from build123d import *

# Parameters (mm, degrees)
F0_R     = 19.05
F1_DEPTH = 50.8
F0_R_2   = 6.857792
F2_DEPTH = 19.05
F3_DEPTH = 19.05
F0_R_3   = 12.7
F4_DEPTH = 38.1


with BuildPart() as f1:
    # F0 (on Top) → F1 (new body)
    with BuildSketch(Plane.XY):
        with BuildLine():
            ThreePointArc((29.102578, -12.692613), (31.081098, -6.482887), (31.75, 0))
            ThreePointArc((31.75, 0), (31.080701, 6.484792), (29.101022, 12.696182))
            ThreePointArc((29.101022, 12.696182), (-0.00495, 31.75), (-29.10498, 12.687106))
            ThreePointArc((-29.10498, 12.687106), (-31.75, -0.005082), (-29.100917, -12.696423))
            ThreePointArc((-29.100917, -12.696423), (0.002078, -31.75), (29.102578, -12.692613))
        make_face()
        Circle(F0_R, mode=Mode.SUBTRACT)
    extrude(amount=F1_DEPTH)

    # F0 (on Top) → F2 (join)
    with BuildSketch(Plane.XY):
        with BuildLine():
            ThreePointArc((-29.100917, -12.696423), (-31.75, -0.005082), (-29.10498, 12.687106))
            Line((-29.10498, 12.687106), (-58.254777, 12.687106))
            Line((-58.254777, 12.687106), (-59.399047, 12.687106))
            ThreePointArc((-59.399047, 12.687106), (-71.52619, -0.135445), (-59.128318, -12.696423))
            Line((-59.128318, -12.696423), (-58.525507, -12.696423))
            Line((-58.525507, -12.696423), (-29.100917, -12.696423))
        make_face()
        with Locations((-58.826912, 0)):
            Circle(F0_R_2, mode=Mode.SUBTRACT)
    extrude(amount=F2_DEPTH)

    # F0 (on Top) → F3 (join)
    with BuildSketch(Plane.XY):
        with BuildLine():
            ThreePointArc((29.101022, 12.696182), (31.080701, 6.484792), (31.75, 0))
            ThreePointArc((31.75, 0), (31.081098, -6.482887), (29.102578, -12.692613))
            Line((29.102578, -12.692613), (74.115909, -12.692613))
            Line((74.115909, -12.692613), (74.982091, -12.692613))
            ThreePointArc((74.982091, -12.692613), (87.248854, 0.060869), (74.860406, 12.696182))
            Line((74.860406, 12.696182), (74.237594, 12.696182))
            Line((74.237594, 12.696182), (29.101022, 12.696182))
        make_face()
        with BuildLine():
            ThreePointArc((74.548989, 6.858), (81.407, -0.000503), (74.547984, -6.858))
            Line((74.547984, -6.858), (46.607984, -6.853861))
            ThreePointArc((46.607984, -6.853861), (39.512576, -0.106876), (46.394271, 6.857956))
            Line((46.394271, 6.857956), (74.548989, 6.858))
        make_face(mode=Mode.SUBTRACT)
    extrude(amount=F3_DEPTH)

    # F0 (on Top) → F4 (join)
    with BuildSketch(Plane.XY):
        Circle(F0_R)
        Circle(F0_R_3, mode=Mode.SUBTRACT)
    extrude(amount=F4_DEPTH)


solid = f1.part
Read the model definition and answer for the solid it produces. Units are mm, in the model's axes. A direction names the side the tool comes from. Coordinates: 2 decimals unless noted, no trailing zeros. Write each loop counter-clockwise with the first axis right and the second up, starting at its lowest first coordinate (ties: lowest second). Pieces come first, ordered by that corner, then holes. Notation, with made-up numbers: (11.5, 1) -> (29.5, 1) arc R21 ccw to (29.5, 18) -> close; hole circle Ø1 at (23, 8). An arc over 180 degrees is marked (long way). Return JSON: item names as keys, results as strings.
(1) Consider line 1 along Y through (x, z) = (0, 44); line 2 along Y through (x, z) = (47, 18.5); line 3 along Z through (x, y) = (-53, -6.5). Determine where each line is inside the solid, lowest interval first. Write a range as from..to.
Answers below:
{"line 1": "-31.75..-19.05, 19.05..31.75", "line 2": "-12.69..-6.85, 6.86..12.7", "line 3": "0..19.05"}
(2) The part is cut by section B-B on z = 28. Give the vertices of the cut face in (x, y).
Answers below:
{"outline": "(29.1, -12.69) arc R31.75 ccw to (31.75, 0) arc R31.75 ccw to (29.1, 12.7) arc R31.75 ccw (long way) to start; hole circle Ø25.4 at (0, 0)"}
(3) Each of these flat-tipped pins is pushed along its axis until it touches: P1, Ø21, axis at x = -44, z = 10, coming from the -Y side; P2, Ø9.5, axis at x = -37.5, z = 13.5, coming from the +Y side; P3, Ø5, axis at x = -45, y = 0.5, coming from the +Z side; P4, Ø1, axis at x = 9, y = -11.5, coming from the -Z side. Where does it stop, or does it pass through?
Answers below:
{"P1": "y = -12.7", "P2": "y = 12.69", "P3": "z = 19.05", "P4": "z = 0"}
(4) The part is cut by section D-D on y = -10. Give the vertices of the cut face in (x, z), then the cut area to 3 significant figures.
Answers below:
{"outline": "(-66.66, 0) -> (-7.83, 0) -> (-7.83, 38.1) -> (-16.21, 38.1) -> (-16.21, 50.8) -> (-30.13, 50.8) -> (-30.13, 19.05) -> (-66.66, 19.05) -> close; (7.83, 0) -> (82.38, 0) -> (82.38, 19.05) -> (30.13, 19.05) -> (30.13, 50.8) -> (16.21, 50.8) -> (16.21, 38.1) -> (7.83, 38.1) -> close", "area": "3,740 mm^2"}
(5) Which of the six approach directions +Z, -Z, +X, -X, +Y, -Y give full straight-line access (tool end or side, diameter ignored) to faces 4 (the cylindrical face through (39.517, -0.259, 9.392)), 5 (the flat face through (-44, 12.687, 9)), 6 (the flat face through (52, 12.696, 9)), 7 (the cylindrical face through (-15.12, -11.59, 44.36))?
Answers below:
{"face 4": "+Z, -Z", "face 5": "+Z, -Z, -X, +Y", "face 6": "+Z, -Z, +X, +Y", "face 7": "+Z"}
(6) The part is cut by section C-C on z = 12. Give the vertices of the cut face in (x, y).
Answers below:
{"outline": "(-59.4, 12.69) arc R12.7 ccw to (-59.13, -12.7) -> (-29.1, -12.7) arc R31.75 ccw to (29.1, -12.69) -> (74.98, -12.69) arc R12.7 ccw to (74.86, 12.7) -> (29.1, 12.7) arc R31.75 ccw to (-29.1, 12.69) -> close; hole circle Ø13.72 at (-58.83, 0); hole circle Ø25.4 at (0, 0); hole (46.39, 6.86) arc R6.86 ccw (long way) to (46.61, -6.85) -> (74.55, -6.86) arc R6.86 ccw to (74.55, 6.86) -> close"}
(7) For a pull along X with two mould halves and no side action, classify faces 1 (the cylindrical face through (-2.75, -12.4, 18.78)), 2 (the flat face through (-11, -7, 0)), 3 (the cylindrical face through (-71.526, 0.138, 9.392)) as pulls with the +X half, pulls with the -X half, needs draft (parallel to the pull), parting line crosses it, or undercut.
Answers below:
{"face 1": "undercut", "face 2": "needs draft", "face 3": "pulls with the -X half"}
(8) The part is cut by section A-A on x = 0. Give the vertices of the cut face in (y, z).
Answers below:
{"outline": "(-31.75, 0) -> (-12.7, 0) -> (-12.7, 38.1) -> (-19.05, 38.1) -> (-19.05, 50.8) -> (-31.75, 50.8) -> close; (12.7, 0) -> (31.75, 0) -> (31.75, 50.8) -> (19.05, 50.8) -> (19.05, 38.1) -> (12.7, 38.1) -> close"}
